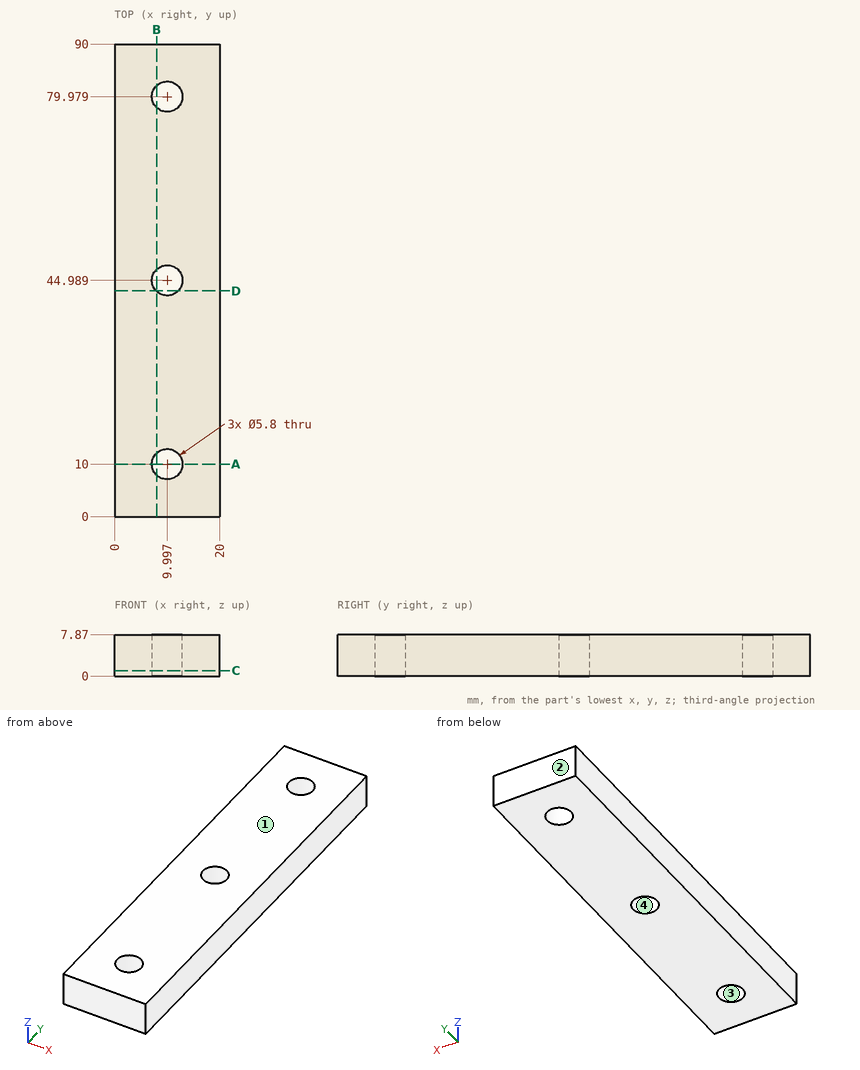
Job drawing, mm, ordinate dimensions from the low corner. One solid piece. Give positions to 0.01 mm unless a question says otherwise; leave off trailing zeros. Loops run counter-clockwise (first coordinate to the right, second up) from the corner with the lowest first, then second, coordinate; pieces in that order, holes last. Notation, with made-up numbers: (70, -9) -> (102, -9) arc R26 cw to (102, 27) -> close; hole circle Ø7 at (68, -34). An arc over 180 degrees is marked (long way). Write each question's results on one line, items separated by ' | '.
(1) Cut at B-B on x = 8. List the corners of the cut face in (y, z) (1 decimal), and give its area (3 significant figures).
Geometry results:
outline: (0, 0) -> (7.9, 0) -> (7.9, 7.9) -> (0, 7.9) -> close; (12.1, 0) -> (42.9, 0) -> (42.9, 7.9) -> (12.1, 7.9) -> close; (47.1, 0) -> (77.9, 0) -> (77.9, 7.9) -> (47.1, 7.9) -> close; (82.1, 0) -> (90, 0) -> (90, 7.9) -> (82.1, 7.9) -> close | area: 609 mm²
(2) Cut at D-D on y = 43. List the corners of the cut face in (x, z).
Geometry results:
outline: (0, 0) -> (7.89, 0) -> (7.89, 7.87) -> (0, 7.87) -> close; (12.11, 0) -> (20, 0) -> (20, 7.87) -> (12.11, 7.87) -> close
(3) Pull direction Y, two halves, no side cores. Call the marked faces 1, 2, 3 and 4: released by +Y, released by -Y, zero draft, split by the parting line, or undercut.
Geometry results:
face 1: zero draft | face 2: released by +Y | face 3: undercut | face 4: undercut
(4) Cut at C-C on z = 1. List the corners of the cut face in (x, y).
Geometry results:
outline: (0, 0) -> (20, 0) -> (20, 90) -> (0, 90) -> close; hole circle Ø5.8 at (10, 10); hole circle Ø5.8 at (10, 44.99); hole circle Ø5.8 at (10, 79.98)
(5) Flat gauge pin, fed straight in: pin 1 Ø5 at (x, y) = (10, 10) entering from +Z. Where does the tip first touch, or does it go through?
Geometry results:
pin 1: passes through
(6) Cut at A-A on y = 10. List the corners of the cut face in (x, z).
Geometry results:
outline: (0, 0) -> (7.1, 0) -> (7.1, 7.87) -> (0, 7.87) -> close; (12.9, 0) -> (20, 0) -> (20, 7.87) -> (12.9, 7.87) -> close
(7) Probe line 1 along Y through (x, z) = (9.75, 4); line 2 along Y through (x, z) = (8.5, 4.5) (1 decimal); line 3 along X through (y, z) = (44, 2.75). List the from-to ranges inside material, lowest first.
Geometry results:
line 1: y = 0 to 7.11, 12.89 to 42.1, 47.88 to 77.09, 82.87 to 90 | line 2: y = 0 to 7.5, 12.5 to 42.5, 47.5 to 77.5, 82.5 to 90 | line 3: x = 0 to 7.27, 12.72 to 20
